Read the model definition and answer for the solid it produces. Units are mm, in the model's axes. Give positions to 0.01 mm unless a question says otherwise; leave off trailing zeros. Order: outer loops, then holes, each group sorted by start corner. A loop starts at its lowest first (then second) coordinate and runs counter-clockwise, first axis right, second up.
```python
from build123d import *

# Parameters (mm, degrees)
SKETCH1_W           = 140
SKETCH1_H           = 100
BOSS_EXTRUDE1_DEPTH = 6.35
SKETCH2_R           = 12.705
SKETCH2_R_2         = 5
CUT_EXTRUDE1_DEPTH  = 10


with BuildPart() as part:
    # Sketch1 → Boss-Extrude1 (new body)
    with BuildSketch(Plane(origin=(0, 0, 0), x_dir=(1, 0, 0), z_dir=(0, 1, 0))):
        with Locations((70, 50)):
            Rectangle(SKETCH1_W, SKETCH1_H)
    extrude(amount=BOSS_EXTRUDE1_DEPTH)

    # Sketch2 → Cut-Extrude1 (cut)
    with BuildSketch(Plane(origin=(0, 6.35, 0), x_dir=(1, 0, 0), z_dir=(0, 1, 0))):
        with Locations(Location((103.75, 30.514428415, 0), (0, 0, 270))):
            Circle(SKETCH2_R)
        with Locations(Location((92.5, 50, 0), (0, 0, 270))):
            Circle(SKETCH2_R_2)
    extrude(amount=-CUT_EXTRUDE1_DEPTH, mode=Mode.SUBTRACT)


solid = part.part
```
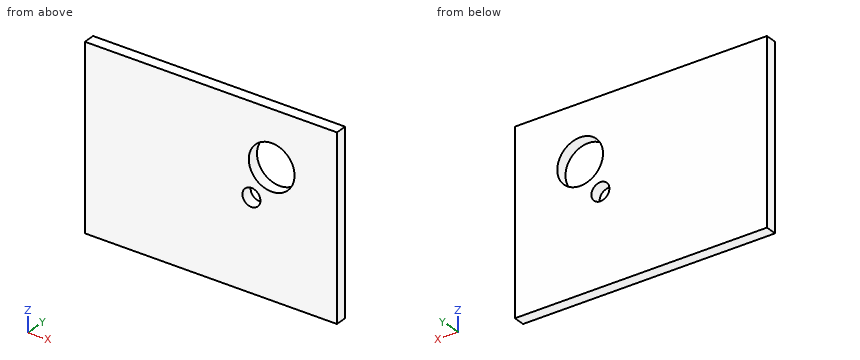
1) The part is cut by section B-B on x = 92.5. Determine the outline of the cut face in (y, z).
Final values:
outline: (0, -100) - (6.35, -100) - (6.35, -55) - (0, -55) - close; (0, -45) - (6.35, -45) - (6.35, -36.42) - (0, -36.42) - close; (0, -24.61) - (6.35, -24.61) - (6.35, 0) - (0, 0) - close
2) The part is cut by section A-A on z = -50. Determine the outline of the cut face in (x, y), and give its area (4 significant figures).
Final values:
outline: (0, 0) - (87.5, 0) - (87.5, 6.35) - (0, 6.35) - close; (97.5, 0) - (140, 0) - (140, 6.35) - (97.5, 6.35) - close
area: 825.5 mm2
3) Consider L1, parallel to X at y = 5, z = -50; L2, parallel to X at y = 1, z = -19.5; L3, parallel to Z at x = 106, y = 2.5. Determine where each line is inside the solid, lowest interval first.
Final values:
L1: x = 0 to 87.5, 97.5 to 140
L2: x = 0 to 97.42, 110.08 to 140
L3: z = -100 to -43.02, -18.01 to 0
4) The part is cut by section C-C on y = 3.75. Determine the outline of the cut face in (x, z) (3 decimals).
Final values:
outline: (0, -100) - (140, -100) - (140, 0) - (0, 0) - close; hole circle Ø10 at (92.5, -50); hole circle Ø25.41 at (103.75, -30.514)
5) The part is cut by section D-D on z = -27. Determine the outline of the cut face in (x, y), and give its area (3 significant figures).
Final values:
outline: (0, 0) - (91.54, 0) - (91.54, 6.35) - (0, 6.35) - close; (115.96, 0) - (140, 0) - (140, 6.35) - (115.96, 6.35) - close
area: 734 mm2
